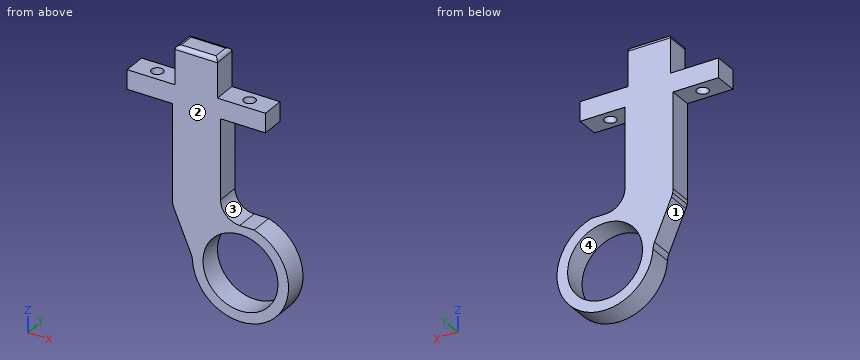
from build123d import *

# Parameters (mm, degrees)
CROQUIS1_R              = 9.75
SALIENTE_EXTRUIR1_DEPTH = 6
CROQUIS2_R              = 1.5
CORTAR_EXTRUIR1_DEPTH   = 6
REDONDEO1_R             = 1


with BuildPart() as part:
    # Croquis1 → Saliente-Extruir1 (new body)
    with BuildSketch(Plane(origin=(0, 0, 0), x_dir=(1, 0, 0), z_dir=(0, 1, 0))):
        with BuildLine():
            Line((-25.374701647, 20.783734094), (-29.767291136, 10.621141392))
            ThreePointArc((-29.767291136, 10.621141392), (-29.942112128, 10.153967486), (-30.069514751, 9.671699501))
            ThreePointArc((-30.069514751, 9.671699501), (-30.150557328, 9.157351254), (-30.17766953, 8.637363805))
            Line((-30.17766953, 8.637363805), (-30.17766953, -16))
            Line((-30.17766953, -16), (-42, -16))
            Line((-42, -16), (-42, -21))
            Line((-42, -21), (-29.5, -21))
            Line((-29.5, -21), (-29.5, -31))
            Line((-29.5, -31), (-18.5, -31))
            Line((-18.5, -31), (-18.5, -21))
            Line((-18.5, -21), (-6, -21))
            Line((-6, -21), (-6, -16))
            Line((-6, -16), (-17.67766953, -16))
            Line((-17.67766953, -16), (-17.67766953, 4.671699501))
            ThreePointArc((-17.67766953, 4.671699501), (-16.213203436, 8.207233407), (-12.67766953, 9.671699501))
            Line((-12.67766953, 9.671699501), (-8.928571429, 9.671699501))
            ThreePointArc((-8.928571429, 9.671699501), (-4.713647249, 31.429321655), (-24.974516609, 22.448404084))
            ThreePointArc((-24.974516609, 22.448404084), (-25.102827296, 21.598812807), (-25.374701647, 20.783734094))
        make_face()
        with Locations((-12.5, 21.650635095)):
            Circle(CROQUIS1_R, mode=Mode.SUBTRACT)
    extrude(amount=SALIENTE_EXTRUIR1_DEPTH)

    # Croquis2 → Cortar-Extruir1 (cut)
    with BuildSketch(Plane.XY.offset(21)):
        with Locations((-36, 3)):
            Circle(CROQUIS2_R)
        with Locations((-12, 3)):
            Circle(CROQUIS2_R)
    extrude(amount=-CORTAR_EXTRUIR1_DEPTH, mode=Mode.SUBTRACT)

    # Redondeo1
    redondeo1_edges = [part.edges().sort_by_distance(p)[0] for p in [
        (-24, 0, 31),
        (-18.5, 3, 31),
        (-29.5, 3, 31),
        (-24, 6, 31),
    ]]
    fillet(redondeo1_edges, radius=REDONDEO1_R)


solid = part.part
Can you work these out from the model? Positions are in its coordinate system, mm. Face numbers are marked on the shaded views. Give positions to 0.01 mm unless a question says otherwise; leave off trailing zeros. Order: outer loops, then holes, each group sorted by start corner. A loop starts at its lowest first (then second) coordinate and runs counter-clockwise, first axis right, second up. Notation, with made-up numbers: M 55.25,-37.75 L 97.25,-37.75 A18 cw 97.25,-24.75 Z; hole C 39.25,-18.5 d5. An arc over 180 degrees is marked long. Use one line per item in the form item = value. Start each with the question number.
Item 1: If we section it at D-D (x = -16): Write out the boundary of the cut face in (y, z).
Item 2: If we section it at B-B (y = 3): Write out the boundary of the cut face in (x, z).
Item 3: If we section it at C-C (z = -13): Write out the boundary of the cut face in (x, y).
Item 4: If we section it at A-A (x = -36): Write out the boundary of the cut face in (y, z), then the cut area to 3 significant figures.
Item 5: If I drill on line 1 along Z through (x, y) = (-12.5, 4.55); line 2 along Z through (x, y) = (-12, 3.25); line 3 along Y through (x, z) = (-36, 18.65), over which ranges is the centre line in solid material (lowest first)?
Item 6: Will these pins go through, and if not, where does the flat tip stop? pin 1 Ø3.5 at (x, y) = (-36, 3) entering from +Z; pin 2 Ø1.8 at (y, z) = (4, 2.5) entering from +X; pin 3 Ø1.8 at (y, z) = (2, 27) entering from +X.
Item 7: We'd pull the mould along Z, two halves only. Please class the marked faces 1, 2, 3 and 4: +Z half, -Z half, draft (parallel to the pull), parting line (faces both ways), or undercut.
Outcome:
q1.outline = M 0,-33.65 L 6,-33.65 L 6,-30.75 L 0,-30.75 Z; M 0,-12.55 L 6,-12.55 L 6,-8.41 L 0,-8.41 Z; M 0,16 L 6,16 L 6,21 L 0,21 Z
q2.outline = M -42,16 L -37.5,16 L -37.5,21 L -42,21 Z; M -34.5,16 L -30.18,16 L -30.18,-8.64 A5 ccw -29.77,-10.62 L -25.37,-20.78 A5 cw -24.97,-22.45 A12.5 ccw long -8.93,-9.67 L -12.68,-9.67 A5 cw -17.68,-4.67 L -17.68,16 L -13.5,16 L -13.5,21 L -18.5,21 L -18.5,30 A1 ccw -19.5,31 L -28.5,31 A1 ccw -29.5,30 L -29.5,21 L -34.5,21 Z; M -10.5,16 L -6,16 L -6,21 L -10.5,21 Z; hole C -12.5,-21.65 d19.5
q3.outline = M -28.74,0 L -17,0 L -17,6 L -28.74,6 Z; M -8,0 L -3.48,0 L -3.48,6 L -8,6 Z
q4.outline = M 0,16 L 1.5,16 L 1.5,21 L 0,21 Z; M 4.5,16 L 6,16 L 6,21 L 4.5,21 Z
q4.area = 15.0 mm2
q5.line_1 = -34.15 to -31.4, -11.9 to -9.67, 16 to 21
q5.line_2 = -34.14 to -31.39, -11.91 to -9.67
q5.line_3 = 0 to 1.5, 4.5 to 6
q6.pin_1 = 21
q6.pin_2 = -17.68
q6.pin_3 = -18.5
q7.face_1 = -Z half
q7.face_2 = draft
q7.face_3 = undercut
q7.face_4 = undercut
